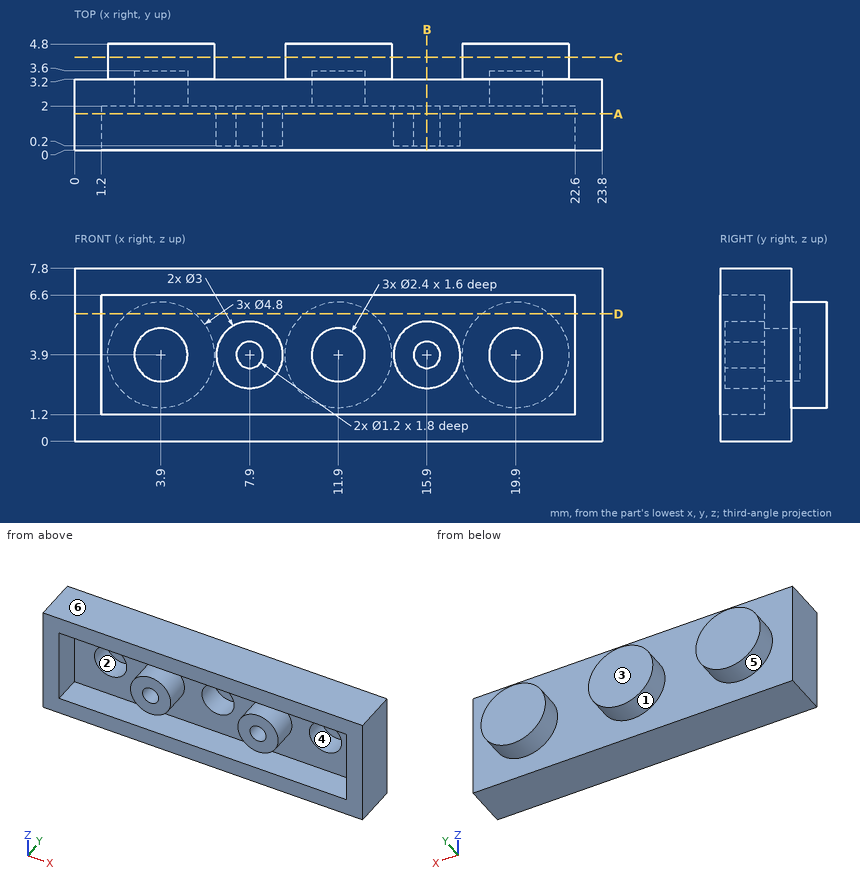
Could you check a few things on this drawing? It's one solid part, dimensions in mm from its lowest x, y, z. A direction names the side the tool comes from. Coordinates: 2 decimals unless noted, no trailing zeros. Write each loop counter-clockwise with the first axis right and the second up, starting at its lowest first coordinate (ties: lowest second). Pieces come first, ordered by that corner, then holes. Notation, with made-up numbers: (5.25, 64.25) - (50.25, 64.25) arc R21 ccw to (50.25, 79.25) - close; hole circle Ø11 at (68, -4). An arc over 180 degrees is marked (long way). Write item = value, one per line.
1) For the marked faces 4, 5 and 6, which set-ups out of +Z, -Z, +X, -X, +Y, -Y let a thin tool reach every point of the face, with its end or its side?
Result set:
face_4 = -Y
face_5 = +Y
face_6 = +Z, +X, -X, +Y, -Y
2) Will these pins go through, and if not, where does the flat tip stop? pin 1 Ø3.5 at (x, z) = (16.5, 3.5) entering from -Y; pin 2 Ø2 at (x, y) = (8, 3.5) entering from +Z; pin 3 Ø2 at (x, z) = (11, 5.5) entering from -Y; pin 4 Ø0.7 at (x, z) = (20.5, 4) entering from -Y.
Result set:
pin_1 = 0.2
pin_2 = 7.8
pin_3 = 2
pin_4 = 3.6
3) Suppose I cut it at C-C on y = 4.2. Please give me the cut outline in (x, z), plus the area to 3 significant figures.
Result set:
outline = circle Ø4.8 at (3.9, 3.9); circle Ø4.8 at (11.9, 3.9); circle Ø4.8 at (19.9, 3.9)
area = 54.3 mm2
4) Suppose I cut it at B-B on x = 15.9. Please give me the cut outline in (y, z), plus the area to 3 significant figures.
Result set:
outline = (0, 0) - (3.2, 0) - (3.2, 7.8) - (0, 7.8) - (0, 6.6) - (2, 6.6) - (2, 5.4) - (0.2, 5.4) - (0.2, 4.5) - (2, 4.5) - (2, 3.3) - (0.2, 3.3) - (0.2, 2.4) - (2, 2.4) - (2, 1.2) - (0, 1.2) - close
area = 17.4 mm2
5) Please list where these lines run through material, in increasing order: line 1 (X direction, y = 3.1, z = 3.9); line 2 (X direction, y = 1.35, z = 3.9); line 3 (X direction, y = 1, z = 1.25). Write a range as [from, to].
Result set:
line_1 = [0, 2.7], [5.1, 10.7], [13.1, 18.7], [21.1, 23.8]
line_2 = [0, 1.2], [6.4, 7.3], [8.5, 9.4], [14.4, 15.3], [16.5, 17.4], [22.6, 23.8]
line_3 = [0, 1.2], [22.6, 23.8]
6) Suppose I cut it at A-A on y = 1.65. Please give me the cut outline in (x, z).
Result set:
outline = (0, 0) - (23.8, 0) - (23.8, 7.8) - (0, 7.8) - close; circle Ø3 at (7.9, 3.9); circle Ø3 at (15.9, 3.9); hole (1.2, 1.2) - (22.6, 1.2) - (22.6, 6.6) - (1.2, 6.6) - close; hole circle Ø1.2 at (7.9, 3.9); hole circle Ø1.2 at (15.9, 3.9)
7) Suppose I cut it at D-D on z = 5.75. Please give me the cut outline in (x, y), plus the area to 3 significant figures.
Result set:
outline = (0, 0) - (1.2, 0) - (1.2, 2) - (22.6, 2) - (22.6, 0) - (23.8, 0) - (23.8, 3.2) - (21.43, 3.2) - (21.43, 4.8) - (18.37, 4.8) - (18.37, 3.2) - (13.43, 3.2) - (13.43, 4.8) - (10.37, 4.8) - (10.37, 3.2) - (5.43, 3.2) - (5.43, 4.8) - (2.37, 4.8) - (2.37, 3.2) - (0, 3.2) - close
area = 48.0 mm2
8) We'd pull the mould along Z, two halves only. Please class the marked faces 1, 2 and 3: +Z half, -Z half, draft (parallel to the pull), parting line (faces both ways), or undercut.
Result set:
face_1 = parting line
face_2 = undercut
face_3 = draft
